Source: CAD feature listing. Evaluate the final solid. Frame: model axes, mm. A direction names the side the tool comes from. Give positions to 0.01 mm unless a question says otherwise; leave off trailing zeros. Order: outer loops, then holes, each group sorted by start corner. A loop starts at its lowest first (then second) coordinate and runs counter-clockwise, first axis right, second up. Notation, with made-up numbers: (57, 49.25) - (85, 49.25) arc R24 cw to (85, 71.25) - close; hole circle Ø5 at (26.25, -32). An arc over 180 degrees is marked (long way). Answer as CSV lines item,"result".
Autodesk Inventor part; units mm, degrees
ref_plane "YZ Plane" through (0, 0, 0) normal (1, 0, 0) x (0, 1, 0)
ref_plane "XZ Plane" through (0, 0, 0) normal (0, 1, 0) x (-1, 0, 0)
ref_plane "XY Plane" through (0, 0, 0) normal (0, 0, 1) x (1, 0, 0)
sketch "Sketch1" plane through (0, 0, 0) normal (0, 0, 1) x (1, 0, 0)
  circle A0 centre (0, 0) radius 6.35
  dimension "d0" = 12.7
extrude "Extrusion1" add sketch "Sketch1" against normal blind 69.85
sketch "Sketch6" plane through (0, 0, 0) normal (0, 0, 1) x (1, 0, 0)
  circle A0 centre (0, 0) radius 6.35
  circle A1 centre (0, 0) radius 2.413
  circle A2 centre (0, 0) radius 4.7625
  dimension "d43" = 4.826
  dimension "d44" = 9.525
extrude "Extrusion11" cut sketch "Sketch6" against normal blind 3.175 contours A0
sketch "Sketch7" plane through (0, 0, -69.85) normal (0, 0, -1) x (-1, 0, 0)
  circle A0 centre (0, 0) radius 6.35
  circle A1 centre (0, 0) radius 4.7625
extrude "Extrusion12" cut sketch "Sketch7" against normal blind 3.175
extrude "Extrusion13" cut sketch "Sketch6" against normal through all contours A1
thread "Thread7"
properties part number "lower box weel shaft steel 2"
(1) Cut plane C-C (z = -22.5). Return loops of the section in (x, y).
Completed:
outline,"circle Ø12.7 at (0, 0); hole circle Ø4.83 at (0, 0)"
(2) Cut plane D-D (y = 4). Return loops of the section in (x, z) (3 decimals), then the cut area to 3 significant figures.
Completed:
outline,"(-4.932, -66.675) - (-2.585, -66.675) - (-2.585, -69.85) - (2.585, -69.85) - (2.585, -66.675) - (4.932, -66.675) - (4.932, -3.175) - (2.585, -3.175) - (2.585, 0) - (-2.585, 0) - (-2.585, -3.175) - (-4.932, -3.175) - close"
area,"659 mm²"
(3) Ray query, line 1 (Y direction, x = 0, z = -51.5); line 2 (Z direction, x = -4.75, y = -4) (3 decimals); line 3 (Y direction, x = -1, z = -54.5). Return the intervals inside material, ascending. Write a range as from..to.
Completed:
line 1,"-6.35..-2.41, 2.41..6.35"
line 2,"-66.675..-3.175"
line 3,"-6.27..-2.2, 2.2..6.27"
(4) Contact query for flat-ended pins moving along their axis: pin 1 (2 mm diameter, centred on y = -3, z = -17.5, fed in from +X); pin 2 (4.5 mm diameter, centred on x = 0, y = 0, fed in from +Z); pin 3 (5 mm diameter, centred on y = 3.5, z = -15.5, fed in from -X); pin 4 (1 mm diameter, centred on x = 1.5, z = -22.5, fed in from +Y). Output: stop coordinate, or through.
Completed:
pin 1,"x = 6.03"
pin 2,"through"
pin 3,"x = -6.27"
pin 4,"y = 6.27"
(5) Access query for faces 1 (the cylindrical face through (-3.78, -2.9, -1.57)), 2 (the flat face through (2, -2, -69.85)), 3 (the cylindrical face through (3.78, -2.9, -68.28)). Directions: +Z, -Z, +X, -X, +Y, -Y. A direction counts if a zero-diameter tool reaches every point of the face in a straight line with its end or side. Return the directions, or none.
Completed:
face 1,"+Z"
face 2,"-Z, +X, -X, +Y, -Y"
face 3,"-Z"
